Print and shaded views of the part. All mm, measured from the part's lowest x, y and z. A direction names the side the tool comes from. Round coordinates to 2 decimals unless told otherwise and drop trailing zeros. Order: outer loops, then holes, each group sorted by start corner. A loop starts at its lowest first (then second) coordinate and runs counter-clockwise, first axis right, second up. Notation, with made-up numbers: M -3.5,64 L 5.5,64 A29 ccw 5.5,92 Z; hole C 40.25,-14 d3. An arc over 180 degrees is marked long. Use CSV: the item, a comma, the result in double quotes.
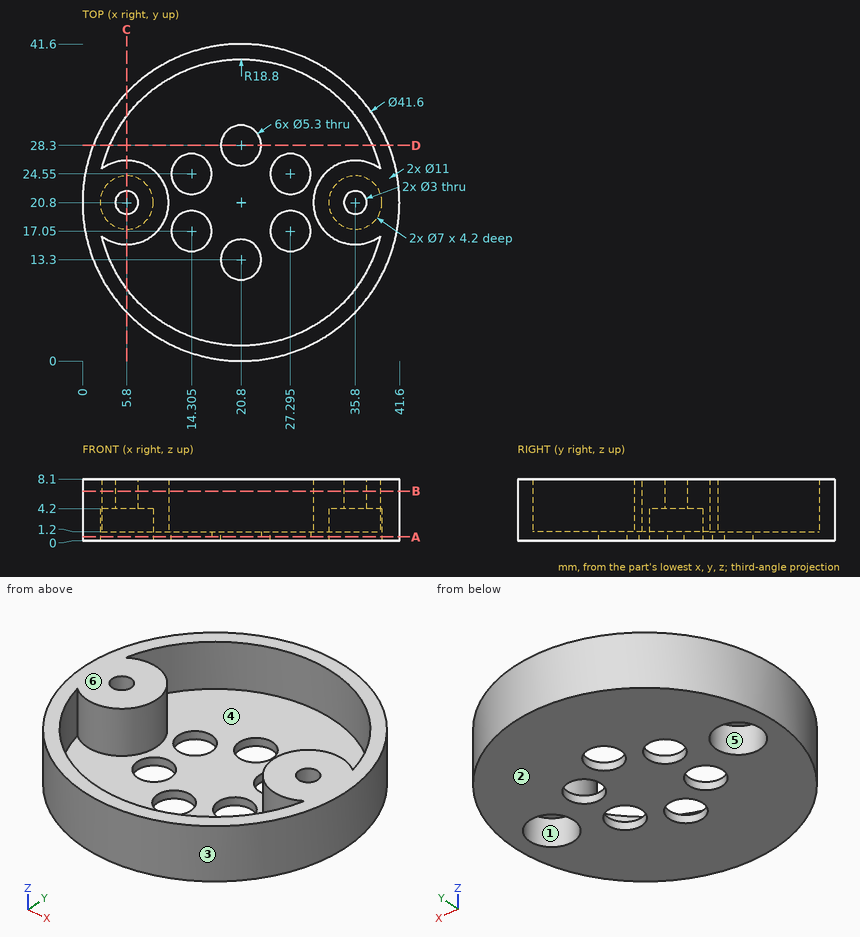
(1) Cut at A-A, the plane z = 0.5. Count the separate pieces of the cut face and the enclosed holes in it, and give its area (3 significant figures).
Answer block:
separate pieces,"1"
enclosed holes,"8"
area,"1,150 mm²"
(2) Drop flat-ended pins along their axis: pin 1 (12 mm diameter, centred on x = 31.5, y = 26.5, fed in from -Z); pin 2 (5 mm diameter, centred on x = 14.3, y = 24.55, fed in from -Z); pin 3 (2 mm diameter, centred on x = 4, y = 21, fed in from -Z); pin 4 (1.5 mm diameter, centred on y = 27, z = 4, fed in from +X). Give the stop position or say it passes through.
Answer block:
pin 1,"stops at z = 0"
pin 2,"passes through"
pin 3,"stops at z = 4.2"
pin 4,"stops at x = 40.87"
(3) Tool access for the marked faces 4, 5 and 6: list every direction of +Z, -Z, +X, -X, +Y, -Y with a clear straight run to the whole face (end or side of a thin tool).
Answer block:
face 4,"+Z"
face 5,"-Z"
face 6,"+Z, +X, -X, +Y, -Y"
(4) Cut at B-B, the plane z = 6.5. Give the cut face in (x, y).
Answer block:
outline,"C 20.8,20.8 d41.6; hole M 2.53,16.38 A18.8 ccw 39.07,16.38 A5.5 cw long 39.07,25.22 A18.8 ccw 2.53,25.22 A5.5 cw long Z; hole C 5.8,20.8 d3; hole C 35.8,20.8 d3"
(5) Two-plate mould, pull along Y, no slides. Class the marked faces 1, 2 and 3: released by +Y, released by -Y, zero draft, split by the parting line, or undercut.
Answer block:
face 1,"undercut"
face 2,"zero draft"
face 3,"split by the parting line"
(6) Cut at D-D, the plane y = 28.3. Give the cut face in (x, z).
Answer block:
outline,"M 1.4,0 L 18.15,0 L 18.15,1.2 L 3.56,1.2 L 3.56,8.1 L 1.4,8.1 Z; M 23.45,0 L 40.2,0 L 40.2,8.1 L 38.04,8.1 L 38.04,1.2 L 23.45,1.2 Z"
(7) Wall check: line 1 (Y direction, x = 20.8, z = 0.8); line 2 (Y direction, x = 36.5, z = 6.75) (1 decimal); line 3 (Y direction, x = 35.8, z = 7.05). Give the ranges that are in metal, low to high. Write a range as from..to.
Answer block:
line 1,"y = 0..10.65, 15.95..25.65, 30.95..41.6"
line 2,"y = 7.2..10.5, 15.3..19.5, 22.1..26.3, 31.1..34.4"
line 3,"y = 6.39..9.47, 15.3..19.3, 22.3..26.3, 32.13..35.21"
(8) Cut at C-C, the plane x = 5.8. Give the cut face in (y, z).
Answer block:
outline,"M 6.39,0 L 17.3,0 L 17.3,4.2 L 19.3,4.2 L 19.3,8.1 L 15.3,8.1 L 15.3,1.2 L 9.47,1.2 L 9.47,8.1 L 6.39,8.1 Z; M 22.3,4.2 L 24.3,4.2 L 24.3,0 L 35.21,0 L 35.21,8.1 L 32.13,8.1 L 32.13,1.2 L 26.3,1.2 L 26.3,8.1 L 22.3,8.1 Z"
